For this review, take the finished solid that the model builds, in its own axes (mm). A direction names the side the tool comes from. Round coordinates to 2 decimals unless told otherwise and drop trailing zeros. Loops run counter-clockwise (first coordinate to the right, second up) from the corner with the lowest first, then second, coordinate; pieces in that order, holes last. Notation, with made-up numbers: (79.5, -6.75) -> (109.5, -6.75) arc R11 ccw to (109.5, 1.25) -> close; hole circle Ø8 at (79.5, 37.5). An arc over 180 degrees is marked (long way). One line per question, with ' | ' between items. Start each with the question number.
1. Wall thickness on line 1 along X through (y, z) = (23.5, 19.5); line 2 along X through (y, z) = (-1.8, 0); line 3 along Y through (x, z) = (61, 20): over which ranges is each line inside the solid? List them lowest first.
2. Consider section D-D (y = 5.5). Write out the cut boundary in (x, z) (3 decimals), and give its area (3 significant figures).
3. Consider section B-B (x = 0). Write out the cut boundary in (y, z) (1 decimal), and give its area (3 significant figures).
4. Consider section A-A (y = 19). Write out the cut boundary in (x, z), and give its area (3 significant figures).
5. For faces 1 (the face through (52, 11, 0)), 2 (the face through (-7.75, -2.46, -1.72)), 3 (the face through (-10.648, -4.93, 13.887)), 4 (the face through (8, 9, -7)), list the 3-axis set-ups (+Z, -Z, +X, -X, +Y, -Y) from which the entire face can be reached by the end or side of a thin tool; tool diameter is ignored.
6. Draft analysis for pull direction Y (two halves, no side actions). For faces 5 (the face through (37, 29, 0)), 6 (the face through (-27.15, 4.56, 26.99)), 7 (the face through (37.465, 19.121, 17.253)), state which applies: pulls with the +Y half, pulls with the -Y half, needs draft (parallel to the pull), parting line crosses it, or undercut.
7. For pin 1 Ø10 at (y, z) = (23, -1.5) entering from -X; pin 2 Ø4.5 at (y, z) = (19, -20) entering from +X; pin 3 Ø18 at (x, z) = (1, -5.5) entering from +Y; pin 4 Ø6.5 at (x, z) = (55, -3) entering from +Y, all flat-tipped, find the tip position at first contact; note any pin that passes through.
```python
from build123d import *

# Parameters (mm, degrees)
SKETCH1_W            = 95
SKETCH1_H            = 60
BOSS_EXTRUDE1_DEPTH  = 9
SKETCH5_R            = 17.5
BOSS_EXTRUDE2_DEPTH  = 10
SKETCH6_R            = 7.9375
CUT_EXTRUDE1_DEPTH   = 14
SKETCH8_R            = 9.525
CUT_EXTRUDE2_DEPTH   = 9
CUT_EXTRUDE3_REACH   = 76.068
SKETCH9_R            = 3.5
BOSS_EXTRUDE3_START  = -30
SKETCH10_W           = 5
SKETCH10_H           = 20
SKETCH10_W_2         = 4
SKETCH10_H_2         = 5
BOSS_EXTRUDE3_DEPTH  = 60
M5_CLEARANCE_HOLE1_D = 5.5
FILLET1_R            = 5
FILLET2_R            = 2.5
FILLET3_R            = 10
FILLET4_R            = 2.5


with BuildPart() as part:
    # Sketch1 → Boss-Extrude1 (new body)
    with BuildSketch(Plane(origin=(0, 0, 0), x_dir=(1, 0, 0), z_dir=(0, 1, 0))):
        with Locations((17.5, 0)):
            Rectangle(SKETCH1_W, SKETCH1_H)
    extrude(amount=BOSS_EXTRUDE1_DEPTH)

    # Sketch5 → Boss-Extrude2 (add)
    with BuildSketch(Plane.XZ):
        with Locations(Location((0, 0, 0), (0, 0, 270))):
            Circle(SKETCH5_R)
    extrude(amount=BOSS_EXTRUDE2_DEPTH)

    # Sketch6 → Cut-Extrude1 (cut)
    with BuildSketch(Plane(origin=(0, 9, 0), x_dir=(1, 0, 0), z_dir=(0, 1, 0))):
        with Locations(Location((0, 0, 0), (0, 0, 270))):
            Circle(SKETCH6_R)
    extrude(amount=-CUT_EXTRUDE1_DEPTH, mode=Mode.SUBTRACT)

    # Sketch8 → Cut-Extrude2 (cut)
    with BuildSketch(Plane(origin=(0, 9, 0), x_dir=(1, 0, 0), z_dir=(0, 1, 0))):
        with Locations(Location((0, 0, 0), (0, 0, 270))):
            Circle(SKETCH8_R)
    extrude(amount=-CUT_EXTRUDE2_DEPTH, mode=Mode.SUBTRACT)

    # Sketch9 → Cut-Extrude3 (cut, up to next)
    with BuildSketch(Plane.XZ.offset(10), mode=Mode.PRIVATE) as cut_extrude3_sk1:
        with Locations(Location((0, 0, 0), (0, 0, 270))):
            Circle(SKETCH9_R)
    cut_extrude3_tool1 = extrude(cut_extrude3_sk1.sketch, amount=-CUT_EXTRUDE3_REACH, mode=Mode.PRIVATE) & part.part
    add(cut_extrude3_tool1.solids().sort_by_distance((0, -10, 0))[0], mode=Mode.SUBTRACT)

    # Sketch10 → Boss-Extrude3 (add)
    with BuildSketch(Plane.XY.offset(BOSS_EXTRUDE3_START)):
        with Locations((62.5, 19)):
            Rectangle(SKETCH10_W, SKETCH10_H)
        with Locations((37.5, 19)):
            Rectangle(SKETCH10_W, SKETCH10_H)
        with Locations((50, 11.5)):
            Rectangle(SKETCH10_W_2, SKETCH10_H_2)
    extrude(amount=BOSS_EXTRUDE3_DEPTH)

    # M5 Clearance Hole1 (through all)
    with Locations(Plane(origin=(65, 0, 0), x_dir=(0, 0, -1), z_dir=(1, 0, 0))):
        with Locations((-20, 19)):
            m5_clearance_hole1 = Hole(M5_CLEARANCE_HOLE1_D / 2)

    # Mirror1: M5 Clearance Hole1 across plane
    add(m5_clearance_hole1.mirror(Plane.XY), mode=Mode.SUBTRACT)

    # Fillet1
    fillet1_edges = [part.edges().sort_by_distance(p)[0] for p in [
        (62.5, 29, -30),
        (62.5, 29, 30),
        (37.5, 29, -30),
        (37.5, 29, 30),
    ]]
    fillet(fillet1_edges, radius=FILLET1_R)

    # Fillet2
    fillet2_edges = [part.edges().sort_by_distance(p)[0] for p in [
        (50, 14, -30),
        (50, 14, 30),
    ]]
    fillet(fillet2_edges, radius=FILLET2_R)

    # Fillet3
    fillet3_edges = [part.edges().sort_by_distance(p)[0] for p in [
        (-30, 4.5, 30),
        (-30, 4.5, -30),
    ]]
    fillet(fillet3_edges, radius=FILLET3_R)

    # Fillet4
    fillet4_edges = [part.edges().sort_by_distance(p)[0] for p in [
        (35, 9, 0),
    ]]
    fillet(fillet4_edges, radius=FILLET4_R)


solid = part.part
```
Answer block:
1) line 1: x = 35 to 40, 60 to 65 | line 2: x = -17.5 to -7.94, 7.94 to 17.5 | line 3: y = 0 to 16.25, 21.75 to 29
2) outline: (-30, -20) arc R10 ccw to (-20, -30) -> (65, -30) -> (65, 30) -> (-20, 30) arc R10 ccw to (-30, 20) -> close; hole circle Ø19.05 at (0, 0) | area: 5,370 mm2
3) outline: (-10, -17.5) -> (0, -17.5) -> (0, -30) -> (9, -30) -> (9, -9.5) -> (0, -9.5) -> (0, -7.9) -> (-5, -7.9) -> (-5, -3.5) -> (-10, -3.5) -> close; (-10, 3.5) -> (-5, 3.5) -> (-5, 7.9) -> (0, 7.9) -> (0, 9.5) -> (9, 9.5) -> (9, 30) -> (0, 30) -> (0, 17.5) -> (-10, 17.5) -> close | area: 604 mm2
4) outline: (35, -30) -> (40, -30) -> (40, -22.75) -> (35, -22.75) -> close; (35, -17.25) -> (40, -17.25) -> (40, 17.25) -> (35, 17.25) -> close; (35, 22.75) -> (40, 22.75) -> (40, 30) -> (35, 30) -> close; (60, -30) -> (65, -30) -> (65, -22.75) -> (60, -22.75) -> close; (60, -17.25) -> (65, -17.25) -> (65, 17.25) -> (60, 17.25) -> close; (60, 22.75) -> (65, 22.75) -> (65, 30) -> (60, 30) -> close | area: 490 mm2
5) face 1: +Z, -Z, +Y | face 2: +Y | face 3: -Y | face 4: +Z, -Z, -X, +Y
6) face 5: pulls with the +Y half | face 6: needs draft | face 7: undercut
7) pin 1: stops at x = 35 | pin 2: passes through | pin 3: stops at y = 9 | pin 4: stops at y = 14
